from build123d import *

# Parameters (mm, degrees)
F1_DEPTH = 25.4


with BuildPart() as f1:
    # F0 (on Front) → F1 (new body)
    with BuildSketch(Plane.XZ):
        Polygon((25.4, 43.994091), (0, 0), (127, 0), (101.6, 43.994091), align=None)
        with BuildLine():
            Line((23.088847, -103.911153), (0, -127))
            Line((0, -127), (127, -127))
            Line((127, -127), (103.911153, -103.911153))
            ThreePointArc((103.911153, -103.911153), (63.5, -120.65), (23.088847, -103.911153))
        make_face()
        with BuildLine():
            Line((23.088847, -23.088847), (0, 0))
            Line((0, 0), (0, -127))
            Line((0, -127), (23.088847, -103.911153))
            ThreePointArc((23.088847, -103.911153), (6.35, -63.5), (23.088847, -23.088847))
        make_face()
        with BuildLine():
            Line((127, -127), (127, 0))
            Line((127, 0), (103.911153, -23.088847))
            ThreePointArc((103.911153, -23.088847), (116.299715, -41.629642), (120.65, -63.5))
            ThreePointArc((120.65, -63.5), (116.299715, -85.370358), (103.911153, -103.911153))
            Line((103.911153, -103.911153), (127, -127))
        make_face()
        with BuildLine():
            Line((25.4, 120.194091), (25.4, 43.994091))
            Line((25.4, 43.994091), (41.04936, 59.64345))
            ThreePointArc((41.04936, 59.64345), (31.75, 82.094091), (41.04936, 104.544731))
            Line((41.04936, 104.544731), (25.4, 120.194091))
        make_face()
        with BuildLine():
            Line((85.95064, 59.64345), (101.6, 43.994091))
            Line((101.6, 43.994091), (101.6, 120.194091))
            Line((101.6, 120.194091), (85.95064, 104.544731))
            ThreePointArc((85.95064, 104.544731), (92.833175, 94.244289), (95.25, 82.094091))
            ThreePointArc((95.25, 82.094091), (92.833175, 69.943892), (85.95064, 59.64345))
        make_face()
        with BuildLine():
            Line((127, 0), (0, 0))
            Line((0, 0), (23.088847, -23.088847))
            ThreePointArc((23.088847, -23.088847), (63.5, -6.35), (103.911153, -23.088847))
            Line((103.911153, -23.088847), (127, 0))
        make_face()
        with BuildLine():
            Line((41.04936, 59.64345), (25.4, 43.994091))
            Line((25.4, 43.994091), (101.6, 43.994091))
            Line((101.6, 43.994091), (85.95064, 59.64345))
            ThreePointArc((85.95064, 59.64345), (63.5, 50.344091), (41.04936, 59.64345))
        make_face()
        with BuildLine():
            Line((101.6, 120.194091), (25.4, 120.194091))
            Line((25.4, 120.194091), (41.04936, 104.544731))
            ThreePointArc((41.04936, 104.544731), (63.5, 113.844091), (85.95064, 104.544731))
            Line((85.95064, 104.544731), (101.6, 120.194091))
        make_face()
    extrude(amount=F1_DEPTH)


solid = f1.part
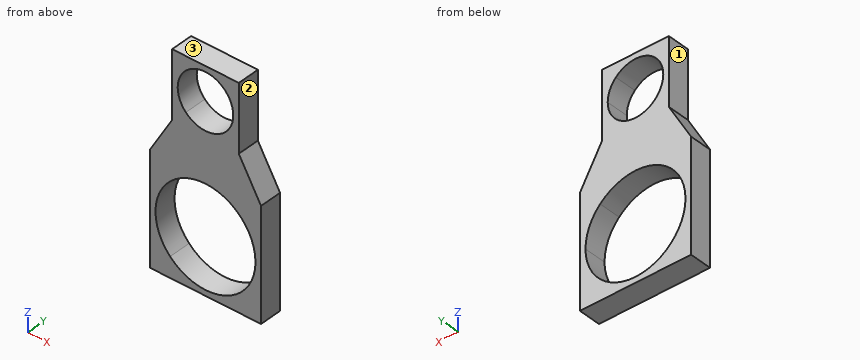
Geometry: final body of the model. Coordinates: model frame, mm. Face numbers are marked on the shaded views. A direction names the side the tool comes from. Give positions to 0.01 mm unless a question says otherwise; leave off trailing zeros. Order: outer loops, then holes, each group sorted by start corner. A loop starts at its lowest first (then second) coordinate and runs counter-clockwise, first axis right, second up. Notation, with made-up numbers: (67.25, 1.5) - (125.25, 1.5) arc R12 cw to (125.25, 18.5) - close; hole circle Ø3 at (62.25, -8.5). An arc over 180 degrees is marked (long way). Use CSV: the item, a comma, the result in double quotes.
1. Access query for the marked faces 1, 2 and 3. Directions: +Z, -Z, +X, -X, +Y, -Y. A direction counts if a zero-diameter tool reaches every point of the face in a straight line with its end or side. Return the directions, or none.
Answers below:
face 1,"+Z, -X, +Y, -Y"
face 2,"+Z, +X, +Y, -Y"
face 3,"+Z, +X, -X, +Y, -Y"
2. Section query B-B (x = 29). Output: boundary loops of the cut face in (y, z).
Answers below:
outline,"(-25.4, -127) - (0, -127) - (0, -109.06) - (-25.4, -109.06) - close; (-25.4, -17.94) - (0, -17.94) - (0, 120.19) - (-25.4, 120.19) - close"
3. Section query D-D (x = 46). Output: boundary loops of the cut face in (y, z), plus the area to 3 significant figures.
Answers below:
outline,"(-25.4, -127) - (0, -127) - (0, -117.9) - (-25.4, -117.9) - close; (-25.4, -9.1) - (0, -9.1) - (0, 55.6) - (-25.4, 55.6) - close; (-25.4, 108.59) - (0, 108.59) - (0, 120.19) - (-25.4, 120.19) - close"
area,"2,170 mm2"
4. Section query A-A (y = -9.25). Output: boundary loops of the cut face in (x, z).
Answers below:
outline,"(0, -127) - (127, -127) - (127, 0) - (101.6, 43.99) - (101.6, 120.19) - (25.4, 120.19) - (25.4, 43.99) - (0, 0) - close; hole (23.09, -103.91) arc R57.15 ccw to (103.91, -103.91) arc R57.15 ccw to (120.65, -63.5) arc R57.15 ccw to (103.91, -23.09) arc R57.15 ccw to (23.09, -23.09) arc R57.15 ccw to start; hole (41.05, 59.64) arc R31.75 ccw to (85.95, 59.64) arc R31.75 ccw to (95.25, 82.09) arc R31.75 ccw to (85.95, 104.54) arc R31.75 ccw to (41.05, 104.54) arc R31.75 ccw to start"
5. Section query C-C (z = 70). Output: boundary loops of the cut face in (x, y), plus the area to 3 significant figures.
Answers below:
outline,"(25.4, -25.4) - (34.14, -25.4) - (34.14, 0) - (25.4, 0) - close; (92.86, -25.4) - (101.6, -25.4) - (101.6, 0) - (92.86, 0) - close"
area,"444 mm2"
6. Contact query for flat-ended pins moving along their axis: pin 1 (1 mm diameter, centred on y = -4, z = 13, fed in from +X); pin 2 (10 mm diameter, centred on y = -15, z = 68.5, fed in from +X); pin 3 (12 mm diameter, centred on y = -15.5, z = 21.5, fed in from -X). Output: stop coordinate, or through.
Answers below:
pin 1,"x = 119.78"
pin 2,"x = 101.6"
pin 3,"x = 8.95"
7. Material intervals for line 1 along Z through (x, y) = (65, -5.5); line 2 along Z through (x, y) = (49, -12.25); line 3 along X through (y, z) = (-23.75, -61.5) (3 decimals), sorted ascending. Write a range as from..to.
Answers below:
line 1,"-127..-120.63, -6.37..50.38, 113.81..120.19"
line 2,"-127..-118.78, -8.22..53.85, 110.34..120.19"
line 3,"0..6.385, 120.615..127"
